from build123d import *

# Parameters (mm, degrees)
SM_BASE_FLANGE_1_DEPTH = 80
SKETCH_6_R             = 5.5
CUT_EXTRUDE_1_DEPTH    = 10
SKETCH_7_R             = 15.5
CUT_EXTRUDE_2_DEPTH    = 10
CUT_EXTRUDE_3_DEPTH    = 10


# Sheet-metal steps are written as plain solids
with BuildPart() as part:
    # Sketch 1 → Базовая кромка1 (new, symmetric)
    with BuildSketch(Plane.XY):
        with BuildLine():
            Line((0, 129), (0, 3))
            ThreePointArc((0, 3), (0.878679656, 0.878679656), (3, 0))
            Line((3, 0), (29, 0))
            Line((29, 0), (29, -3))
            Line((29, -3), (3, -3))
            ThreePointArc((3, -3), (-1.242640687, -1.242640687), (-3, 3))
            Line((-3, 3), (-3, 129))
            Line((-3, 129), (0, 129))
        make_face()
    extrude(amount=SM_BASE_FLANGE_1_DEPTH, both=True)

    # Эскиз6 → Вырез-Вытянуть1 (cut)
    with BuildSketch(Plane(origin=(0, 0, 0), x_dir=(0, 0, -1), z_dir=(1, 0, 0))):
        with Locations(Location((-66, 111, 0), (0, 0, 90))):
            Circle(SKETCH_6_R)
        with Locations(Location((66, 111, 0), (0, 0, 90))):
            Circle(SKETCH_6_R)
        with Locations(Location((66, 61, 0), (0, 0, 90))):
            Circle(SKETCH_6_R)
        with Locations(Location((-66, 61, 0), (0, 0, 90))):
            Circle(SKETCH_6_R)
    extrude(amount=-CUT_EXTRUDE_1_DEPTH, mode=Mode.SUBTRACT)

    # Эскиз7 → Вырез-Вытянуть2 (cut)
    with BuildSketch(Plane(origin=(0, 0, 0), x_dir=(0, 0, -1), z_dir=(1, 0, 0))):
        with Locations(Location((-45, 38, 0), (0, 0, 90))):
            Circle(SKETCH_7_R)
        with Locations(Location((45, 38, 0), (0, 0, 90))):
            Circle(SKETCH_7_R)
    extrude(amount=-CUT_EXTRUDE_2_DEPTH, mode=Mode.SUBTRACT)

    # Эскиз8 → Вырез-Вытянуть3 (cut)
    with BuildSketch(Plane(origin=(0, 0, 0), x_dir=(1, 0, 0), z_dir=(0, 1, 0))):
        with BuildLine():
            Line((16, -43.5), (29, -43.5))
            ThreePointArc((29, -43.5), (35.5, -50), (29, -56.5))
            Line((29, -56.5), (16, -56.5))
            ThreePointArc((16, -56.5), (9.5, -50), (16, -43.5))
        make_face()
        with BuildLine():
            Line((16, 56.5), (29, 56.5))
            ThreePointArc((29, 56.5), (35.5, 50), (29, 43.5))
            Line((29, 43.5), (16, 43.5))
            ThreePointArc((16, 43.5), (9.5, 50), (16, 56.5))
        make_face()
    extrude(amount=-CUT_EXTRUDE_3_DEPTH, mode=Mode.SUBTRACT)


solid = part.part
Could you check a few things on this model? Use its own coordinates, in mm. A direction names the side the tool comes from. Round coordinates to 2 decimals unless told otherwise and drop trailing zeros. Order: outer loops, then holes, each group sorted by start corner. A loop starts at its lowest first (then second) coordinate and runs counter-clockwise, first axis right, second up. Notation, with made-up numbers: M 54.5,-2.75 L 66.5,-2.75 A11 cw 66.5,8.25 Z; hole C 17,-38 d1. An arc over 180 degrees is marked long. One line per item, written item: value.
(1) I need wall thicknesses on line 1 along Z through (x, y) = (-0.8, 38); line 2 along Z through (x, y) = (-1.7, 111); line 3 along X through (y, z) = (22.5, 16.5). Which ranges of each line are inside material? Lowest first, please. Write a range as from..to.
Ans:
line 1: z = -80..-60.5, -29.5..29.5, 60.5..80
line 2: z = -80..-71.5, -60.5..60.5, 71.5..80
line 3: x = -3..0
(2) Imagine slicing it at D-D (z = -8.5). Write out the boundary of the cut face in (x, y).
Ans:
outline: M -3,3 A6 ccw 3,-3 L 29,-3 L 29,0 L 3,0 A3 cw 0,3 L 0,129 L -3,129 Z
(3) I'm going to push flat-ended pins straight in: P1, Ø1.5, axis at y = 48.5, z = -14, coming from the +X side; P2, Ø1, axis at x = 18, z = 20.5, coming from the +Y side. Where does each tip first touch, or does it pass through?
Ans:
P1: stops at x = 0
P2: stops at y = 0
(4) Which directions (+Z, -Z, +X, -X, +Y, -Y) give clear straight access to the entire face, cutting with the end or side of a thin tool? Please do faces 1 (the cylindrical face through (-1.479, 52.784, -40.344)), 2 (the flat face through (0, 67, 1)).
Ans:
face 1: +X, -X
face 2: +Z, -Z, +X, +Y
(5) Imagine slicing it at B-B (x = 25). Write out the boundary of the cut face in (y, z), and give its area (3 significant figures).
Ans:
outline: M -3,-80 L 0,-80 L 0,-56.5 L -3,-56.5 Z; M -3,-43.5 L 0,-43.5 L 0,43.5 L -3,43.5 Z; M -3,56.5 L 0,56.5 L 0,80 L -3,80 Z
area: 402 mm^2
(6) If we mould it in two halves opening along Y, with no side actions, what happens to faces 3 (the flat face through (-1, 44, -80)), 4 (the flat face through (16, 0, 1)), 5 (the cylindrical face through (-1.48, 46.33, 58.07)), 6 (the cylindrical face through (-1.479, 105.505, -65.758))? For each: released by +Y, released by -Y, zero draft, split by the parting line, or undercut.
Ans:
face 3: zero draft
face 4: released by +Y
face 5: undercut
face 6: undercut
(7) Imagine slicing it at C-C (z = -32). Write out the boundary of the cut face in (x, y).
Ans:
outline: M -3,3 A6 ccw 3,-3 L 29,-3 L 29,0 L 3,0 A3 cw 0,3 L 0,29.56 L -3,29.56 Z; M -3,46.44 L 0,46.44 L 0,129 L -3,129 Z
(8) Imagine slicing it at A-A (y = 38). Write out the boundary of the cut face in (x, z), and give its area (3 significant figures).
Ans:
outline: M -3,-80 L 0,-80 L 0,-60.5 L -3,-60.5 Z; M -3,-29.5 L 0,-29.5 L 0,29.5 L -3,29.5 Z; M -3,60.5 L 0,60.5 L 0,80 L -3,80 Z
area: 294 mm^2
